Work out the finished part from the listing and answer in its coordinate system (mm). A direction names the side the tool comes from. Coordinates: 2 decimals unless noted, no trailing zeros. Write each loop counter-clockwise with the first axis right and the second up, starting at its lowest first coordinate (ties: lowest second). Pieces come first, ordered by that corner, then holes. Notation, with made-up numbers: M -26.5,75.25 L 8.5,75.25 A19 ccw 8.5,80.25 Z; hole C -20.75,-1.5 d7. An arc over 180 degrees is marked long. Answer as CSV lines item,"result". Start each with the question number.
(1) A cutting plane is placed at D-D on z = 2.45. Count the separate pieces of the cut face and the enclosed holes in it, then the cut area to 3 significant figures.
(2) Find the intervals of material crossed by L1, parallel to Y at x = -12.5, z = 0.95; L2, parallel to Y at x = 5.5, z = 4; L3, parallel to Y at x = -5, z = 1.25, in increasing order. Write a range as [from, to].
(3) A cutting plane is placed at C-C on x = -9. Give the vertices of the cut face in (y, z).
(4) For faces 4 (the flat face through (-5.455, 27, 3)), 5 (the flat face through (-12.106, 24, 3)), 6 (the flat face through (-4, 27, 5.8)), determine the directions among +Z, -Z, +X, -X, +Y, -Y from which every point of the face is accessible in a straight line to the end or side of a thin tool.
(5) Flat-ended cylindrical pins translate along their axes: P1, Ø1.5, axis at y = 30, z = 3, coming from the -X side; P2, Ø2, axis at x = 1.5, y = 37, coming from the -Z side; P3, Ø2.5, axis at y = 24, z = 4, coming from the -X side. Find the tip coordinate at first contact, or state that the pin passes through.
(6) The mould has two halves that part along Y. Classify faces 1 (the flat face through (-1, 44.084, 3)), 2 (the flat face through (-17.786, 37, 3)), 3 (the flat face through (-11, 29.357, 3)): released by +Y, released by -Y, zero draft, split by the parting line, or undercut.
(7) A cutting plane is placed at A-A on x = -3.5. Give the vertices of the cut face in (y, z).
(8) A cutting plane is placed at B-B on x = -15.5. Give the vertices of the cut face in (y, z), then the cut area to 3 significant figures.
from build123d import *

# Parameters (mm, degrees)
SKETCH1_RX          = 8.334694939
SKETCH1_RY          = 8.1
SKETCH1_W           = 27.929114048
SKETCH1_H           = 3.401184302
SKETCH1_H_2         = 3.401184301
BOSS_EXTRUDE1_DEPTH = 5.8


with BuildPart() as part:
    # Sketch1 → Boss-Extrude1 (new body)
    with BuildSketch(Plane.XY):
        Polygon((-5.45496555, 25.036590129), (-5.45496555, 28.132290129), (-9.705575673, 28.132290129), (-9.705575673, 29.356690129), (-12.105575673, 29.356690129), (-12.105575673, 28.132290129), (-14.605575673, 28.132290129), (-14.605575673, 31.084440129), (-17.785575673, 31.084440129), (-17.785575673, 44.084440129), (17.214424327, 44.084440129), (17.214424327, 9.084440129), (-17.785575673, 9.084440129), (-17.785575673, 22.084440129), (-14.785575673, 22.084440129), (-14.785575673, 25.036590129), (-12.105575673, 25.036590129), (-12.105575673, 23.812190129), (-9.705575673, 23.812190129), (-9.705575673, 25.036590129), align=None)
        with Locations((5.879729388, 26.584440129)):
            Ellipse(SKETCH1_RX, SKETCH1_RY, mode=Mode.SUBTRACT)
        with Locations((0.120011131, 39.38503228)):
            Rectangle(SKETCH1_W, SKETCH1_H, mode=Mode.SUBTRACT)
        with Locations((0.120011131, 13.783847979)):
            Rectangle(SKETCH1_W, SKETCH1_H_2, mode=Mode.SUBTRACT)
    extrude(amount=BOSS_EXTRUDE1_DEPTH)


solid = part.part
Here are the results:
1,separate pieces,"1"
1,enclosed holes,"3"
1,area,"761 mm^2"
2,L1,"y = [9.08, 12.08], [15.48, 25.04], [28.13, 37.68], [41.09, 44.08]"
2,L2,"y = [9.08, 12.08], [15.48, 18.49], [34.68, 37.68], [41.09, 44.08]"
2,L3,"y = [9.08, 12.08], [15.48, 37.68], [41.09, 44.08]"
3,outline,"M 9.08,0 L 12.08,0 L 12.08,5.8 L 9.08,5.8 Z; M 15.48,0 L 25.04,0 L 25.04,5.8 L 15.48,5.8 Z; M 28.13,0 L 37.68,0 L 37.68,5.8 L 28.13,5.8 Z; M 41.09,0 L 44.08,0 L 44.08,5.8 L 41.09,5.8 Z"
4,face 4,"+Z, -Z, -X"
4,face 5,"+Z, -Z"
4,face 6,"+Z, +X, -X, +Y, -Y"
5,P1,"stops at x = -14.61"
5,P2,"stops at z = 0"
5,P3,"stops at x = -14.79"
6,face 1,"released by +Y"
6,face 2,"zero draft"
6,face 3,"undercut"
7,outline,"M 9.08,0 L 12.08,0 L 12.08,5.8 L 9.08,5.8 Z; M 15.48,0 L 37.68,0 L 37.68,5.8 L 15.48,5.8 Z; M 41.09,0 L 44.08,0 L 44.08,5.8 L 41.09,5.8 Z"
8,outline,"M 9.08,0 L 22.08,0 L 22.08,5.8 L 9.08,5.8 Z; M 31.08,0 L 44.08,0 L 44.08,5.8 L 31.08,5.8 Z"
8,area,"151 mm^2"
